For this review, take the finished solid that the model builds, in its own axes (mm). Face numbers are marked on the shaded views. A direction names the side the tool comes from. Coordinates: 2 decimals unless noted, no trailing zeros. Write each loop counter-clockwise with the first axis right and the second up, starting at its lowest first coordinate (ties: lowest second). Pieces come first, ordered by that corner, then holes.
1) For the marked faces 4, 5, 6 and 7, list the 3-axis set-ups (+Z, -Z, +X, -X, +Y, -Y) from which the entire face can be reached by the end or side of a thin tool; tool diameter is ignored.
2) Mouldability with a two-part tool opening along X and no side actions: class the marked faces 1, 2 and 3 as pulls with the +X half, pulls with the -X half, needs draft (parallel to the pull), parting line crosses it, or undercut.
3) We need section A-A on y = 4. Write out the cut boundary in (x, z), then the cut area to 3 significant figures.
4) Insertion check: P1, Ø5, axis at x = -4, y = 5.5, coming from the -Z side; P2, Ø3.5, axis at x = -5.5, y = 4.5, coming from the +Z side; P3, Ø1, axis at x = -3.5, z = -6, coming from the +Y side; P4, Ø8, axis at x = 4, z = 4, coming from the +Y side. Each pin has a flat end and moves straight along its axis. Give the tip position at first contact, or say it passes through.
5) To check wall thickness, follow line 1 along X through (y, z) = (6.65, 0); line 2 along Z through (x, y) = (6.3, 4); line 3 along X through (y, z) = (2.75, 1). State the ranges of each line that lie inside material, in increasing order.
Autodesk Inventor part; units mm, degrees
ref_plane "Work Plane2" through (8, -4, 0) normal (0, -1, 0) x (0, 0, 1)
ref_plane "YZ Plane" through (0, 0, 0) normal (1, 0, 0) x (0, 1, 0)
ref_plane "XZ Plane" through (0, 0, 0) normal (0, 1, 0) x (-1, 0, 0)
sketch "Sketch1" plane through (0, 0, 0) normal (0, 1, 0) x (-1, 0, 0)
  line L0 (-8, 0) -> (-8, 8)
  line L1 (-8, 8) -> (8, 8)
  line L2 (8, 8) -> (8, -8)
  line L3 (8, -8) -> (-8, -8)
  line L4 (-8, -8) -> (-8, 0)
  circle A0 centre (0, 0) radius 1.5
  line L5 (8, 8) -> (8, 4.5)
  line L6 (8, 4.5) -> (5, 4.5)
  line L7 (-8, 8) -> (-8, 4.5)
  line L8 (-8, 4.5) -> (-5, 4.5)
  line L9 (0, 0) -> (0, 4.5)
  dimension "d0" = 8
  dimension "d1" = 8
  dimension "d2" = 16
  dimension "d3" = 16
  dimension "d4" = 16
  dimension "d5" = 8
  dimension "d25" = 3
  dimension "d95" = 3.5
  dimension "d96" = 3
  dimension "d106" = 3.5
  dimension "d107" = 3
  dimension "d196" = 4.5
ref_plane "Work Plane2" through (8, -4, 0) normal (0, -1, 0) x (0, 0, 1)
sketch "Sketch3" plane through (8, -4, 0) normal (0, -1, 0) x (0, 0, 1)
  line L0 (5.5, 8) -> (5.5, 7)
  line L1 (5.5, 7) -> (3.5, 7)
  line L2 (3.5, 7) -> (3.5, 9)
  line L3 (3.5, 9) -> (5.5, 9)
  line L4 (5.5, 9) -> (5.5, 8)
  line L5 (0, 8) -> (3.5, 8)
  dimension "d16" = 1
  dimension "d17" = 2
  dimension "d18" = 2
  dimension "d19" = 2
  dimension "d20" = 1
  dimension "d27" = 3.5
loft "Loft1" add profiles "Sketch1", "Sketch3" contours L0 L1 L2 L3 L4 | A0 / all
sketch "Sketch5" plane through (-8, 0, -8) normal (0, 1, 0) x (1, 0, 0)
  line L0 (8, -8) -> (8, -12.5)
  circle A0 centre (8, -12.5) radius 0.5
  dimension "d28" = 4.5
  dimension "d29" = 1
hole "Hole1" at (0, 0, 4.5) direction (0, -1, 0) diameter 1 depth 4
sketch "Sketch6" plane through (-8, 0, -8) normal (0, 1, 0) x (1, 0, 0)
  line L0 (8, -8) -> (10.8, -8)
  line L1 (16, 0) -> (16, -16)
  line L2 (10.8, -8) -> (10.8, -6)
  line L3 (10.8, -6) -> (15.3, -6)
  line L4 (15.3, -6) -> (15.3, -10)
  line L5 (15.3, -10) -> (10.8, -10)
  line L6 (10.8, -10) -> (10.8, -8)
  line L7 (15.3, -8) -> (16, -8)
  dimension "d180" = 2
  dimension "d181" = 4.5
  dimension "d182" = 4
  dimension "d183" = 4.5
  dimension "d184" = 2
  dimension "d185" = 0.7
  dimension "d197" = 2.8
extrude "Extrusion1" add sketch "Sketch6" along normal blind 8.5
sketch "Sketch7" plane through (-8, 8.5, -8) normal (0, 1, 0) x (1, 0, 0)
  line L0 (8, -8) -> (13.5, -8)
  circle A0 centre (13.5, -8) radius 0.5
  circle A1 centre (13.5, -8) radius 0.75
  dimension "d48" = 5.5
  dimension "d49" = 1
  dimension "d57" = 1.5
hole "Hole2" at (5.5, 8.5, 0) direction (0, -1, 0) diameter 1 depth 2.5
sketch "Sketch8" plane through (-8, 0, -8) normal (0, 1, 0) x (1, 0, 0)
  line L0 (8, -8) -> (5.2, -8)
  line L1 (5.2, -8) -> (5.2, -6)
  line L2 (5.2, -6) -> (0.7, -6)
  line L3 (0.7, -6) -> (0.7, -10)
  line L4 (0.7, -10) -> (5.2, -10)
  line L5 (5.2, -10) -> (5.2, -8)
  line L6 (0.7, -8) -> (0, -8)
  dimension "d58" = 2.8
  dimension "d59" = 2
  dimension "d60" = 4.5
  dimension "d61" = 4
  dimension "d62" = 4.5
  dimension "d63" = 2
  dimension "d179" = 0.7
extrude "Extrusion2" add sketch "Sketch8" along normal blind 8.5
sketch "Sketch9" plane through (-8, 8.5, -8) normal (0, 1, 0) x (1, 0, 0)
  line L0 (8, -8) -> (2.5, -8)
  circle A0 centre (2.5, -8) radius 0.5
  circle A1 centre (2.5, -8) radius 0.75
  dimension "d66" = 5.5
  dimension "d67" = 1
  dimension "d75" = 1.5
hole "Hole3" at (-5.5, 8.5, 0) direction (0, -1, 0) diameter 1 depth 2.5
sketch "Sketch11" plane through (-7.3, 0, -2) normal (-1, 0, 0) x (0, 0, 1)
  line L0 (2, 0) -> (2, 4)
  circle A0 centre (2, 4) radius 0.5
  dimension "d85" = 4
  dimension "d86" = 1
hole "Hole5" at (-7.3, 4, 0) direction (1, 0, 0) diameter 1 depth 1.5
sketch "Sketch13" plane through (-8, 0, -8) normal (-0.4961389, -0.8682431, 0) x (0.8682431, -0.4961389, 0)
  line L0 (0, 16) -> (0, 0)
  line L1 (0, 16) -> (0, 12.5)
  line L2 (0, 12.5) -> (4, 12.5)
  circle A0 centre (4, 12.5) radius 0.25
  point P0 (6.9459, 8)
  dimension "d97" = 3.5
  dimension "d98" = 0.5
  dimension "d118" = 4
hole "Hole6" at (-4.527, -1.9846, 4.5) direction (0.4961389, 0.8682431, 0) diameter 1 depth 1
sketch "Sketch14" plane through (8, 0, -8) normal (0.4961389, -0.8682431, 0) x (0.8682431, 0.4961389, 0)
  line L0 (0, 16) -> (-8.0623, 13.5)
  line L1 (0, 16) -> (0, 12.5)
  line L2 (0, 0) -> (0, 16)
  line L3 (0, 12.5) -> (-4, 12.5)
  circle A0 centre (-4, 12.5) radius 0.25
  point P0 (-6.9459, 8)
  dimension "d108" = 3.5
  dimension "d109" = 0.5
  dimension "d117" = 4
hole "Hole7" at (4.527, -1.9846, 4.5) direction (-0.4961389, 0.8682431, 0) diameter 1 depth 1
sketch "Sketch15" plane through (-8, 0, -8) normal (0, -0.9444968, -0.3285206) x (1, 0, 0)
  line L0 (0, 0) -> (16, 0)
  line L1 (0, 0) -> (8, 0)
  line L2 (8, 0) -> (8, 8.4687)
  circle A0 centre (8, 8.4687) radius 0.25
  dimension "d119" = 8
  dimension "d120" = 0.5
hole "Hole8" at (0, -2.7821, -0.0014) direction (0, 0.9444968, 0.3285206) diameter 1 depth 1
sketch "Sketch17" plane through (-8, 0, -8) normal (0, 1, 0) x (1, 0, 0)
  line L0 (8, -8) -> (8, -3.5)
  circle A0 centre (8, -3.5) radius 0.25
  dimension "d128" = 4.5
  dimension "d129" = 0.5
hole "Hole9" at (0, 0, -4.5) direction (0, -1, 0) diameter 1 depth 3
sketch "Sketch21" plane through (-8, 0, -8) normal (0, 1, 0) x (1, 0, 0)
  circle A0 centre (8, -8) radius 0.8
  dimension "d171" = 1.6
hole "Hole12" at (0, 0, 0) direction (0, -1, 0) diameter 1.8 depth 0.6
sketch "Sketch22" plane through (7.3, 0, 2) normal (1, 0, 0) x (0, 0, -1)
  line L0 (2, 0) -> (2, 4)
  line L1 (2, 0) -> (6, 0) construction
  circle A0 centre (2, 4) radius 0.5
  dimension "d186" = 4
  dimension "d187" = 90
  dimension "d188" = 1
hole "Hole13" at (7.3, 4, 0) direction (-1, 0, 0) diameter 1 depth 1.5
sketch "Sketch23" plane through (-8, 0, -8) normal (0, 1, 0) x (1, 0, 0)
  line L0 (15.3, -10) -> (10.8, -10)
  line L1 (15.3, -10) -> (15.3, -15)
  point P0 (8, -8)
  dimension "d198" = 5
ref_plane "Work Plane" through (8, 0, 0) normal (0, -1, 0) x (0, 0, 1)
properties material "ABS Plastic"
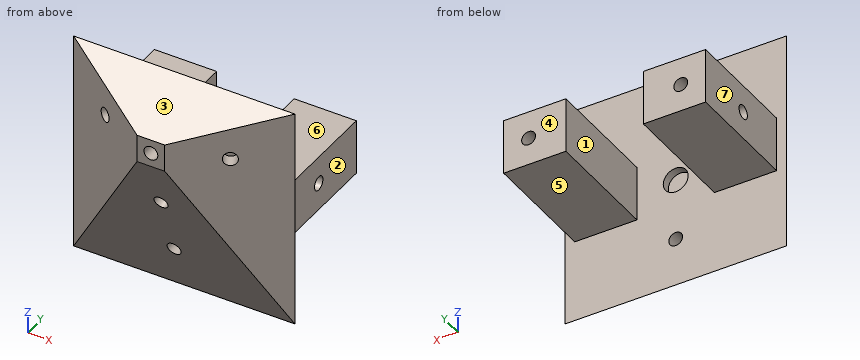
Result:
1. face 4: +Z, -Z, +X, -X, +Y
1. face 5: -Z, +X, -X, +Y
1. face 6: +Z, +X, -X, +Y
1. face 7: +Z, -Z, -X, +Y
2. face 1: undercut
2. face 2: pulls with the +X half
2. face 3: needs draft
3. outline: (-7.3, -2) - (-2.8, -2) - (-2.8, 2) - (-7.3, 2) - (-7.3, 0.5) - (-5.8, 0.5) - (-5.8, -0.5) - (-7.3, -0.5) - close; (2.8, -2) - (7.3, -2) - (7.3, -0.5) - (5.8, -0.5) - (5.8, 0.5) - (7.3, 0.5) - (7.3, 2) - (2.8, 2) - close
3. area: 33.0 mm2
4. P1: stops at z = -2
4. P2: stops at z = 2
4. P3: stops at y = 0
4. P4: stops at y = 8.5
5. line 1: x = -7.3 to -6, -5 to -2.8, 2.8 to 5, 6 to 7.3
5. line 2: z = -2 to -0.5, 0.5 to 2
5. line 3: x = -7.3 to -2.8, 2.8 to 7.3
